Design review of the part shown in the three views and the two pictorial views. Dimensions are in mm from the part's minimum x, y and z. Give positions to 0.01 mm unless a question says otherwise; leave off trailing zeros. Write each loop counter-clockwise with the first axis right and the second up, starting at its lowest first coordinate (ties: lowest second). Pieces come first, ordered by that corner, then holes.
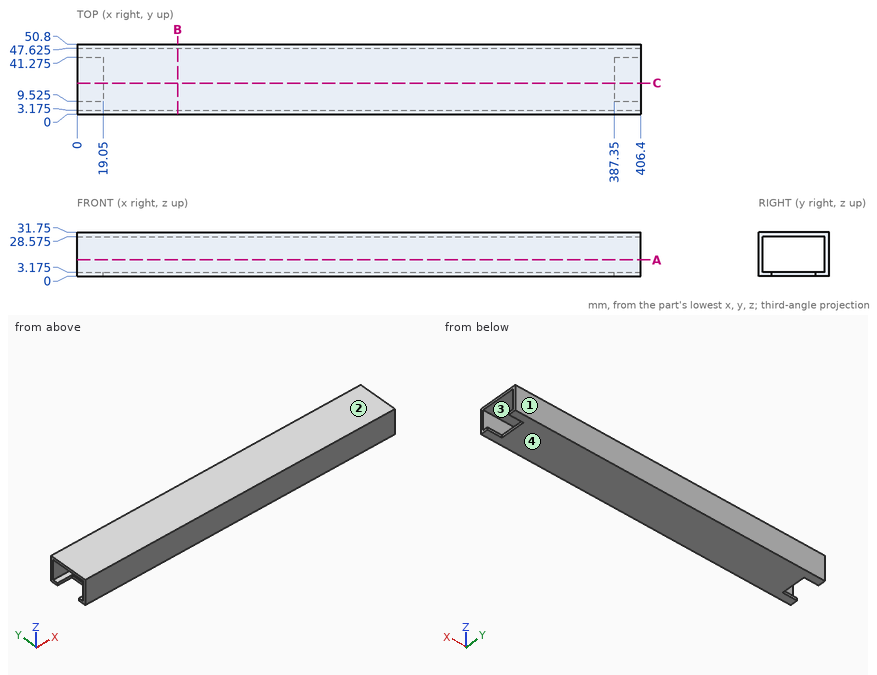
(1) To check wall thickness, follow L1, parallel to Y at x = 236, z = 18 (3 decimals); L2, parallel to Z at x = 192, y = 36.5 (3 decimals). State the ranges of each line that lie inside material, in increasing order.
Resolved:
L1: y = 0 to 3.175, 47.625 to 50.8
L2: z = 0 to 3.175, 28.575 to 31.75
(2) Consider section A-A, the plane z = 12. Give the boundary of the cut face in (x, y) (3 decimals).
Resolved:
outline: (0, 0) - (406.4, 0) - (406.4, 3.175) - (0, 3.175) - close; (0, 47.625) - (406.4, 47.625) - (406.4, 50.8) - (0, 50.8) - close
(3) Consider section B-B, the plane x = 72.5. Give the boundary of the cut face in (y, z) (3 decimals).
Resolved:
outline: (0, 0) - (50.8, 0) - (50.8, 31.75) - (0, 31.75) - close; hole (3.175, 3.175) - (47.625, 3.175) - (47.625, 28.575) - (3.175, 28.575) - close
(4) Clearance check with flat-ended pins moving along their axes: P1, Ø5, axis at y = 41.5, z = 6, coming from the -X side; P2, Ø2, axis at y = 33.5, z = 4, coming from the -X side; P3, Ø1.6, axis at y = 19.5, z = 2, coming from the +X side. State where each tip first meets the part, or that it passes through.
Resolved:
P1: passes through
P2: stops at x = 19.05
P3: stops at x = 387.35
(5) Mouldability with a two-part tool opening along Z and no side actions: class the marked faces 1, 2, 3 and 4 as pulls with the +Z half, pulls with the -Z half, needs draft (parallel to the pull), parting line crosses it, or undercut.
Resolved:
face 1: needs draft
face 2: pulls with the +Z half
face 3: undercut
face 4: pulls with the -Z half
(6) Consider section C-C, the plane y = 22.5. Give the boundary of the cut face in (x, z) (3 decimals), then the cut area to 3 significant figures.
Resolved:
outline: (0, 28.575) - (406.4, 28.575) - (406.4, 31.75) - (0, 31.75) - close; (19.05, 0) - (387.35, 0) - (387.35, 3.175) - (19.05, 3.175) - close
area: 2,460 mm2
